Design review of the part built by this model. Coordinates are the model's own, in mm. A direction names the side the tool comes from. Give positions to 0.01 mm unless a question says otherwise; leave off trailing zeros. Order: outer loops, then holes, each group sorted by start corner. A loop starts at its lowest first (then second) coordinate and runs counter-clockwise, first axis right, second up. Notation, with made-up numbers: M 74.5,-20.5 L 125.5,-20.5 A30 cw 125.5,18.5 Z; hole C 70,-16.5 d5. An arc over 180 degrees is marked long. Put each result on its own line as item: value. Start each with the question number.
from build123d import *

# Parameters (mm, degrees)
BOSS_EXTRUDE2_DEPTH   = 6
BOSS_EXTRUDE2_2_DEPTH = 6
SKETCH1_3_R           = 2.1
BOSS_EXTRUDE3_DEPTH   = 3.8
SKETCH3_R             = 3.1
CUT_EXTRUDE2_DEPTH    = 3


with BuildPart() as part:
    # Sketch1 → Boss-Extrude2 (new body)
    with BuildSketch(Plane(origin=(0, 0, 0), x_dir=(-1, 0, 0), z_dir=(0, 0, 1))):
        Polygon((9.209773359, -16.292309171), (-15.475780333, -28.232378111), (-15.475780333, -34.232378111), (4.947252827, -24.354032787), align=None)
    extrude(amount=-BOSS_EXTRUDE2_DEPTH)



with BuildPart() as body_2:
    # Sketch1 → Boss-Extrude2 2 (new body)
    with BuildSketch(Plane(origin=(0, 0, 0), x_dir=(-1, 0, 0), z_dir=(0, 0, 1))):
        with BuildLine():
            Line((-16.475780333, -11.132378111), (11.93801277, -11.132378111))
            Line((11.93801277, -11.132378111), (13.524219667, -8.132378111))
            ThreePointArc((13.524219667, -8.132378111), (13.580869915, -6.628117273), (13.750499733, -5.132378111))
            Line((13.750499733, -5.132378111), (-16.475780333, -5.132378111))
            Line((-16.475780333, -5.132378111), (-16.475780333, -11.132378111))
        make_face()
    extrude(amount=-BOSS_EXTRUDE2_2_DEPTH)


with BuildPart() as part_1:
    add(part.part)

    add(body_2.part)  # Boss-Extrude3 merges body 2
    # Sketch1_3 → Boss-Extrude3 (add)
    with BuildSketch(Plane(origin=(0, 0, 0), x_dir=(-1, 0, 0), z_dir=(0, 0, 1))):
        with BuildLine():
            Line((-15.475780333, -28.232378111), (-15.475780333, -34.232378111))
            Line((-15.475780333, -34.232378111), (28.470653106, -12.976081758))
            ThreePointArc((28.470653106, -12.976081758), (40.434092032, -7.012706779), (27.199664346, -5.132378111))
            Line((27.199664346, -5.132378111), (-16.475780333, -5.132378111))
            Line((-16.475780333, -5.132378111), (-16.475780333, -11.132378111))
            Line((-16.475780333, -11.132378111), (19.877697964, -11.132378111))
            Line((19.877697964, -11.132378111), (-15.475780333, -28.232378111))
        make_face()
        with Locations(Location((33.524219667, -8.132378111, 0), (0, 0, 180))):
            Circle(SKETCH1_3_R, mode=Mode.SUBTRACT)
    extrude(amount=-BOSS_EXTRUDE3_DEPTH)

    # Sketch3 → Cut-Extrude2 (cut)
    with BuildSketch(Plane(origin=(0, 0, -3.8), x_dir=(-1, 0, 0), z_dir=(0, 0, -1))):
        with Locations((33.524219667, 8.132378111)):
            Circle(SKETCH3_R)
    extrude(amount=-CUT_EXTRUDE2_DEPTH, mode=Mode.SUBTRACT)


solid = part_1.part
1. To check wall thickness, follow probe 1 along Z at (x, y) = (-27.5, 10); probe 2 along Y at (x, z) = (-3, -3.9); probe 3 along Y at (x, z) = (7, -1.55). State the ranges of each line that lie inside material, in increasing order.
2. Consider section D-D on y = 18. Give the boundary of the cut face in (x, z).
3. The part is to be moulded in two halves that separate along X. For faces 1 (the cylindrical face through (-35.191, 6.855, -0.394)), 2 (the flat face through (-6, 5.132, -3)), 3 (the flat face through (-12.72, 9.65, -4.88)), 4 (the flat face through (-36, 7, -0.8)), say which applies: +X half, -X half, draft (parallel to the pull), parting line (faces both ways), or undercut.
4. Consider section A-A on z = -5.2. Give the boundary of the cut face in (x, y).
5. Consider section B-B on x = -33. Give the boundary of the cut face in (y, z).
6. Consider section C-C on z = -2.1. Give the boundary of the cut face in (x, y).
7. Machinability: for faces 5 (the flat face through (16.476, 8, -3)), 6 (the cylindrical face through (-36.39, 6.95, -2.32)), 7 (the flat face through (2, 8, -6)), 8 (the flat face through (15.476, 31, -3)), 9 (the cylindrical face through (-13.58, 6.65, -4.88)), which of the approach directions +Z, -Z, +X, -X, +Y, -Y give a long, thin tool a straight path to every point of the face, cutting with its end or side? Answer none if there is none.
8. Insertion check: pin 1 (3 mm diameter, centred on x = -15.5, z = -2.5, fed in from -Y); pin 2 (3 mm diameter, centred on y = 26.5, z = -2, fed in from +X); pin 3 (3 mm diameter, centred on y = 12, z = -2.5, fed in from -X). Each pin has a flat end and moves straight along its axis. Give the tip position at first contact, or say it passes through.
Returned:
1. probe 1: z = -3.8 to 0
1. probe 2: y = 5.13 to 11.13, 19.3 to 25.3
1. probe 3: y = 5.13 to 11.13, 24.13 to 30.13
2. outline: M -18.08,-3.8 L -8.31,-3.8 L -8.31,-6 L -5.68,-6 L -5.68,0 L -18.08,0 Z
3. face 1: undercut
3. face 2: draft
3. face 3: -X half
3. face 4: undercut
4. outline: M -13.75,5.13 L 16.48,5.13 L 16.48,11.13 L -11.94,11.13 L -13.52,8.13 A20 cw Z; M -9.21,16.29 L 15.48,28.23 L 15.48,34.23 L -4.95,24.35 Z
5. outline: M 1.15,-3.8 L 5.08,-3.8 L 5.08,-0.8 L 6.1,-0.8 L 6.1,0 L 1.15,0 Z; M 10.17,-0.8 L 11.19,-0.8 L 11.19,-3.8 L 15.11,-3.8 L 15.11,0 L 10.17,0 Z
6. outline: M -28.47,12.98 A7 ccw long -27.2,5.13 L 16.48,5.13 L 16.48,11.13 L -19.88,11.13 L 15.48,28.23 L 15.48,34.23 Z; hole C -33.52,8.13 d6.2
7. face 5: +Z, -Z, +X, +Y, -Y
7. face 6: -Z
7. face 7: -Z, +X, -X, +Y, -Y
7. face 8: +Z, -Z, +X, +Y
7. face 9: -Z, -X, +Y
8. pin 1: stops at y = 5.13
8. pin 2: stops at x = 15
8. pin 3: stops at x = -40.11
